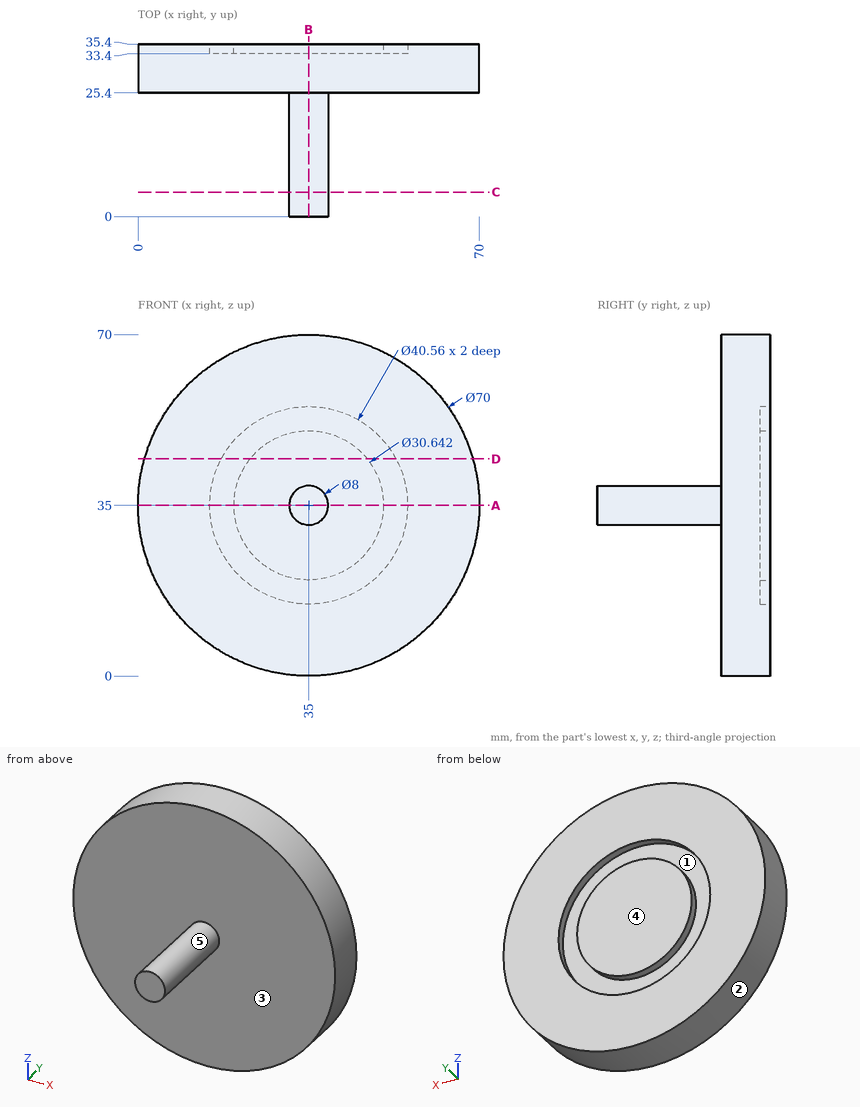
Study the drawing (mm; zero at the part's minimum x, y, z) and answer. A direction names the side the tool comes from. Round coordinates to 2 decimals unless told otherwise and drop trailing zeros. Loops run counter-clockwise (first coordinate to the right, second up) from the corner with the lowest first, then second, coordinate; pieces in that order, holes last. Notation, with made-up numbers: (9.25, 34) - (28.25, 34) arc R4 cw to (28.25, 39) - close; hole circle Ø2 at (-17, 88). An arc over 180 degrees is marked (long way). Use one line per item in the form item = value. Start each with the question number.
1. The part is cut by section B-B on x = 35. Determine the outline of the cut face in (y, z).
2. The part is cut by section C-C on y = 5. Determine the outline of the cut face in (x, z).
3. A tool of negligible diameter and unlimited length cuts with its end or side. For the marked faces 4 and 5, from which of +Z, -Z, +X, -X, +Y, -Y can it reach the whole face along a straight path? Write none if from no direction.
4. The part is cut by section D-D on z = 44.5. Determine the outline of the cut face in (x, y), then the cut area to 3 significant figures.
5. Given pin 1 Ø2 at (y, z) = (30, 52) entering from +X; pin 2 Ø2 at (x, y) = (30, 29.5) entering from +Z; pin 3 Ø6 at (x, y) = (26, 14) entering from +Z; pin 4 Ø1 at (y, z) = (31, 37.5) entering from -X, each flat-ended and moving along its own axis, determine where each tip first touches the part or whether it passes through.
6. The part is cut by section A-A on z = 35. Determine the outline of the cut face in (x, y).
7. For a pull along Z with two mould halves and no side action, classify the marked faces 1, 2 and 3 as pulls with the +Z half, pulls with the -Z half, needs draft (parallel to the pull), parting line crosses it, or undercut.
8. Consider line 1 (Z direction, x = 35, y = 34.95); line 2 (Y direction, x = 10, z = 48). Determine where each line is inside the solid, lowest interval first. Write a range as [from, to].
Geometry check:
q1.outline = (0, 31) - (25.4, 31) - (25.4, 0) - (35.4, 0) - (35.4, 14.72) - (33.4, 14.72) - (33.4, 19.68) - (35.4, 19.68) - (35.4, 50.32) - (33.4, 50.32) - (33.4, 55.28) - (35.4, 55.28) - (35.4, 70) - (25.4, 70) - (25.4, 39) - (0, 39) - close
q2.outline = circle Ø8 at (35, 35)
q3.face_4 = +Z, -Z, +X, -X, +Y
q3.face_5 = -Y
q4.outline = (1.31, 25.4) - (68.69, 25.4) - (68.69, 35.4) - (52.92, 35.4) - (52.92, 33.4) - (47.02, 33.4) - (47.02, 35.4) - (22.98, 35.4) - (22.98, 33.4) - (17.08, 33.4) - (17.08, 35.4) - (1.31, 35.4) - close
q4.area = 650 mm^2
q5.pin_1 = 66.13
q5.pin_2 = 69.77
q5.pin_3 = through
q5.pin_4 = 0.06
q6.outline = (0, 25.4) - (31, 25.4) - (31, 0) - (39, 0) - (39, 25.4) - (70, 25.4) - (70, 35.4) - (55.28, 35.4) - (55.28, 33.4) - (50.32, 33.4) - (50.32, 35.4) - (19.68, 35.4) - (19.68, 33.4) - (14.72, 33.4) - (14.72, 35.4) - (0, 35.4) - close
q7.face_1 = undercut
q7.face_2 = parting line crosses it
q7.face_3 = needs draft
q8.line_1 = [0, 14.72], [19.68, 50.32], [55.28, 70]
q8.line_2 = [25.4, 35.4]
